Source: CAD feature listing. Evaluate the final solid. Frame: model axes, mm. Round coordinates to 2 decimals unless told otherwise and drop trailing zeros. Loops run counter-clockwise (first coordinate to the right, second up) from the corner with the lowest first, then second, coordinate; pieces in that order, holes last. Notation, with made-up numbers: (14.5, 77.5) -> (56.5, 77.5) arc R19 ccw to (56.5, 83.5) -> close; hole circle Ø2 at (22.5, 52.25). An arc over 180 degrees is marked (long way). Put each result on its own line as item: value. Start each with the question number.
1. Draft query along Y for faces 1 (the flat face through (0, -146, -34.925)), 2 (the flat face through (0, 0, 0)), 3 (the cylindrical face through (-0.1, -292.1, 0.1)), 4 (the cylindrical face through (0.13, -319.71, -24.96)). Return one class per face: pulls with the +Y half, pulls with the -Y half, needs draft (parallel to the pull), parting line crosses it, or undercut.
2. Material intervals for L1, parallel to Y at x = -3, z = 1.5; L2, parallel to Y at x = 4, z = 29.5; L3, parallel to Z at x = 7.5, y = -292.5 (3 decimals), sorted ascending.
3. Cut plane A-A (x = 2.5). Return the cut outline in (y, z) (3 decimals).
4. Contact query for flat-ended pins moving along their axis: pin 1 (1 mm diameter, centred on x = -4, z = -25.5, fed in from +Y); pin 2 (1 mm diameter, centred on x = -6.5, z = 17, fed in from -Y); pin 3 (1.5 mm diameter, centred on x = -1.5, z = 26, fed in from -Y). Output: stop coordinate, or through.
```python
from build123d import *

# Parameters (mm, degrees)
F0_W     = 19.05
F0_H     = 69.85
F1_DEPTH = 330.2
F3_D     = 6.35
F5_DEPTH = 19.051
F6_W     = 25.4
F6_H     = 25.4
F7_DEPTH = 304.8


with BuildPart() as f1:
    # F0 (on Front) → F1 (new body)
    with BuildSketch(Plane.XZ):
        Rectangle(F0_W, F0_H)
    extrude(amount=F1_DEPTH)

    # F3 (through all)
    with Locations(Plane.YZ.offset(9.525)):
        with Locations((-295.275, 0)):
            Hole(F3_D / 2)

    # F4 (on face) → F5 (cut, through all)
    with BuildSketch(Plane.YZ.offset(9.525)):
        with BuildLine():
            Line((-330.2, -34.925), (-295.814604, -34.925))
            ThreePointArc((-295.814604, -34.925), (-319.973652, -24.698652), (-330.2, -0.539604))
            Line((-330.2, -0.539604), (-330.2, -34.925))
        make_face()
        with BuildLine():
            Line((-330.2, 34.925), (-330.2, 0.539604))
            ThreePointArc((-330.2, 0.539604), (-319.973652, 24.698652), (-295.814604, 34.925))
            Line((-295.814604, 34.925), (-330.2, 34.925))
        make_face()
    extrude(amount=-F5_DEPTH, mode=Mode.SUBTRACT)


with BuildPart() as f7:
    # F6 (on Front) → F7 (new body)
    with BuildSketch(Plane.XZ):
        with Locations((72.780613, -13.592582)):
            Rectangle(F6_W, F6_H)
    extrude(amount=F7_DEPTH)


solid = f1.part
```
Solution:
1. face 1: needs draft
1. face 2: pulls with the +Y half
1. face 3: undercut
1. face 4: pulls with the -Y half
2. L1: y = -330.17 to -298.07, -292.48 to 0
2. L2: y = -313.98 to 0
2. L3: z = -34.925 to -1.543, 1.543 to 34.925
3. outline: (-330.2, -0.54) arc R34.929 ccw to (-295.815, -34.925) -> (0, -34.925) -> (0, 34.925) -> (-295.815, 34.925) arc R34.929 ccw to (-330.2, 0.54) -> close; hole circle Ø6.35 at (-295.275, 0)
4. pin 1: stops at y = 0
4. pin 2: stops at y = -326.06
4. pin 3: stops at y = -319.41
